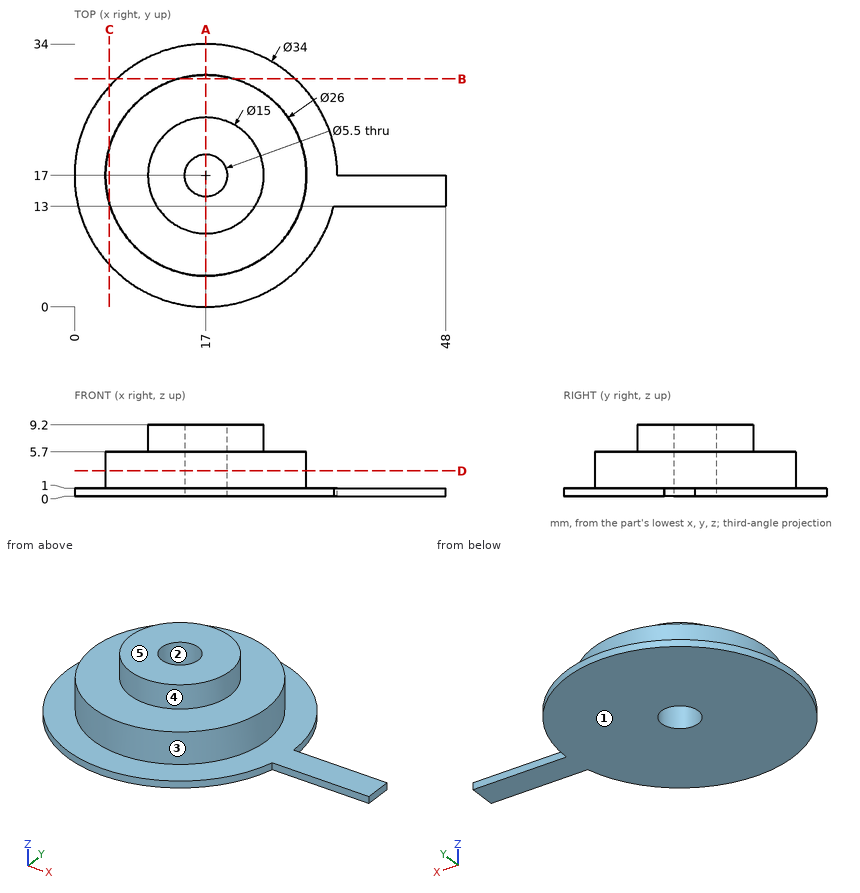
Verification items for this drawing (mm, ordinates from the low corner). A direction names the side the tool comes from. Coordinates: 2 decimals unless noted, no trailing zeros. Write each loop counter-clockwise with the first axis right and the second up, starting at its lowest first coordinate (ties: lowest second). Pieces come first, ordered by that corner, then holes. Notation, with made-up numbers: M -21,-4.5 L 31,-4.5 A25 ccw 31,34.5 Z; hole C -14.75,37 d4. An arc over 180 degrees is marked long. Use CSV: the item, a comma, the result in double quotes.
Q1. Set-up check for the marked faces 4 and 5: record each of +Z, -Z, +X, -X, +Y, -Y from which the full face is reachable in a straight line by a thin tool's end or side.
Computed values:
face 4,"+Z"
face 5,"+Z, +X, -X, +Y, -Y"
Q2. Go/stop test with flat-tipped pins: P1, Ø1.1, axis at x = 38.5, z = 0.5, coming from the +Y side; P2, Ø0.8, axis at x = 39.5, z = 0.5, coming from the -Y side; P3, Ø1, axis at x = 9, z = 6, coming from the +Y side. Record where each tip stops, or that it passes through.
Computed values:
P1,"y = 17"
P2,"y = 13"
P3,"y = 27.55"
Q3. Thickness scan on line 1 along Y through (x, z) = (17, 6.5); line 2 along Y through (x, z) = (17, 3). Record the ranges inside material, lowest first. Write a range as [from, to].
Computed values:
line 1,"[9.5, 14.25], [19.75, 24.5]"
line 2,"[4, 14.25], [19.75, 30]"
Q4. Section check B-B, the plane y = 29.5. Enter the section's corners in (x, z), and give its area (3 significant figures).
Computed values:
outline,"M 5.48,0 L 28.52,0 L 28.52,1 L 20.57,1 L 20.57,5.7 L 13.43,5.7 L 13.43,1 L 5.48,1 Z"
area,"56.6 mm²"
Q5. Mould release check, pull along X, two halves, no side actions. Record for the marked faces 1, 2 and 3: pulls with the +X half, pulls with the -X half, needs draft (parallel to the pull), parting line crosses it, or undercut.
Computed values:
face 1,"needs draft"
face 2,"undercut"
face 3,"parting line crosses it"
Q6. Section check D-D, the plane z = 3.25. Enter the section's corners in (x, y).
Computed values:
outline,"C 17,17 d26; hole C 17,17 d5.5"
Q7. Section check A-A, the plane x = 17. Enter the section's corners in (y, z), and give its area (3 significant figures).
Computed values:
outline,"M 0,0 L 14.25,0 L 14.25,9.2 L 9.5,9.2 L 9.5,5.7 L 4,5.7 L 4,1 L 0,1 Z; M 19.75,0 L 34,0 L 34,1 L 30,1 L 30,5.7 L 24.5,5.7 L 24.5,9.2 L 19.75,9.2 Z"
area,"158 mm²"
